from build123d import *

# Parameters (mm, degrees)
FACE_2_DEPTH            = 5
SKETCH2_W               = 14.632926246
SKETCH2_H               = 5
BOSS_EXTRUDE2_DEPTH     = 7
SKETCH3_W               = 14.632926246
SKETCH3_H               = 7
BOSS_EXTRUDE3_DEPTH     = 7
EYE_HOLES_REACH         = 248.075
SKETCH4_R               = 1.15
SKETCH5_W               = 14.632926246
SKETCH5_H               = 3.5
SEAT_DEPTH              = 7
SKETCH6_W               = 18
SKETCH6_H               = 5
BOSS_EXTRUDE4_DEPTH     = 3.5
SKETCH7_W               = 18.025006546
SKETCH7_H               = 4.25
TOP_HOLE_DEPTH          = 248.972829901
MIDDLE_HOLE_DEPTH       = 246.672789516
MIDDLE_HOLE_DEPTH_BACK  = 246.672789516
SKETCH8_R               = 5.003684601
CUT_EXTRUDE8_DEPTH      = 208.598432106
CUT_EXTRUDE8_DEPTH_BACK = 3.5
SKETCH10_R              = 1.15
SKETCH11_R              = 0.754398486
CUT_EXTRUDE9_DEPTH      = 246.672789516


with BuildPart() as part:
    # Sketch1 → Face 2 (new body)
    with BuildSketch(Plane.XY):
        Polygon((189.199131389, 129.336090234), (189.219408928, 129.168352428), (189.276625012, 129.01501095), (189.375109043, 128.870497126), (189.879763338, 128.333185306), (190.417075159, 127.828531011), (190.558185088, 127.731803407), (190.715733881, 127.672634267), (190.882668266, 127.652553357), (205.515594512, 127.652553357), (205.683332318, 127.672830896), (205.84007769, 127.731803407), (205.98118762, 127.828531011), (207.023153735, 128.870497126), (207.118523911, 129.009007135), (207.17885385, 129.168352428), (207.199131389, 129.336090234), (207.199131389, 132.202042434), (189.199131389, 132.202042434), align=None)
    extrude(amount=FACE_2_DEPTH)

    # Sketch2 → Boss-Extrude2 (add)
    with BuildSketch(Plane.XZ.offset(-127.652553357)):
        with Locations((198.199131389, 2.5)):
            Rectangle(SKETCH2_W, SKETCH2_H)
    extrude(amount=BOSS_EXTRUDE2_DEPTH)

    # Sketch3 → Boss-Extrude3 (add)
    with BuildSketch(Plane(origin=(0, 0, 0), x_dir=(-1, 0, 0), z_dir=(0, 0, -1))):
        with Locations((-198.199131389, 124.152553357)):
            Rectangle(SKETCH3_W, SKETCH3_H)
    extrude(amount=BOSS_EXTRUDE3_DEPTH)

    # Sketch4 → Eye Holes (cut, up to next)
    with BuildSketch(Plane.XY.offset(5), mode=Mode.PRIVATE) as eye_holes_sk1:
        with Locations((191.649131389, 129.852042434)):
            Circle(SKETCH4_R)
    eye_holes_tool1 = extrude(eye_holes_sk1.sketch, amount=-EYE_HOLES_REACH, mode=Mode.PRIVATE) & part.part
    # Sketch4 → Eye Holes (cut, up to next)
    with BuildSketch(Plane.XY.offset(5), mode=Mode.PRIVATE) as eye_holes_sk2:
        with Locations((204.599131389, 129.852042434)):
            Circle(SKETCH4_R)
    eye_holes_tool2 = extrude(eye_holes_sk2.sketch, amount=-EYE_HOLES_REACH, mode=Mode.PRIVATE) & part.part
    add(eye_holes_tool1.solids().sort_by_distance((191.649131, 129.852042, 5))[0], mode=Mode.SUBTRACT)
    add(eye_holes_tool2.solids().sort_by_distance((204.599131, 129.852042, 5))[0], mode=Mode.SUBTRACT)

    # Sketch5 → Seat (cut)
    with BuildSketch(Plane(origin=(0, 0, -7), x_dir=(-1, 0, 0), z_dir=(0, 0, -1))):
        with Locations((-198.199131389, 125.902553357)):
            Rectangle(SKETCH5_W, SKETCH5_H)
    extrude(amount=-SEAT_DEPTH, mode=Mode.SUBTRACT)

    # Sketch6 → Boss-Extrude4 (add)
    with BuildSketch(Plane(origin=(0, 132.202042434, 0), x_dir=(1, 0, 0), z_dir=(0, 1, 0))):
        with Locations((198.199131389, -2.5)):
            Rectangle(SKETCH6_W, SKETCH6_H)
    extrude(amount=BOSS_EXTRUDE4_DEPTH)

    # Sketch7 → Top Hole (cut, through all)
    with BuildSketch(Plane.XY.offset(5)):
        with Locations((198.194207579, 133.577042434)):
            Rectangle(SKETCH7_W, SKETCH7_H)
    extrude(amount=-TOP_HOLE_DEPTH, mode=Mode.SUBTRACT)

    # Sketch8 → Middle Hole (cut, two sides: drawn at the far end of the back side and taken through both)
    with BuildSketch(Plane.XY.offset(5).offset(-MIDDLE_HOLE_DEPTH_BACK)):
        with Locations((198.199131389, 131.452042434)):
            Circle(SKETCH8_R)
    extrude(amount=MIDDLE_HOLE_DEPTH + MIDDLE_HOLE_DEPTH_BACK, mode=Mode.SUBTRACT)

    # Sketch10 → Cut-Extrude8 (cut, two sides: drawn at the far end of the back side and taken through both)
    with BuildSketch(Plane.XZ.offset(-120.652553357).offset(-CUT_EXTRUDE8_DEPTH_BACK)):
        with Locations((193.382668266, -3.308334882)):
            Circle(SKETCH10_R)
        with Locations((203.015594512, -3.308334882)):
            Circle(SKETCH10_R)
    extrude(amount=CUT_EXTRUDE8_DEPTH + CUT_EXTRUDE8_DEPTH_BACK, mode=Mode.SUBTRACT)

    # Sketch11 → Cut-Extrude9 (cut, through all)
    with BuildSketch(Plane.XY.offset(5)):
        with Locations((192.88691871, 131.452042434)):
            Circle(SKETCH11_R)
        with Locations((202.919958348, 131.377258625)):
            Circle(SKETCH11_R)
    extrude(amount=-CUT_EXTRUDE9_DEPTH, mode=Mode.SUBTRACT)


solid = part.part
Could you check a few things on this model? Use its own coordinates, in mm. A direction names the side the tool comes from. Coordinates: 2 decimals unless noted, no trailing zeros. Order: outer loops, then holes, each group sorted by start corner. A loop starts at its lowest first (then second) coordinate and runs counter-clockwise, first axis right, second up.
Q1. Suppose I cut it at A-A on x = 191.25. Please give me the cut outline in (y, z).
Q2. Which directions (+Z, -Z, +X, -X, +Y, -Y) give clear straight access to the entire face, cutting with the end or side of a thin tool? Please do faces 5 (the flat face through (198, 126, 0)), 6 (the flat face through (190.883, 123, 0)), 7 (the cylindrical face through (192.234, 122.427, -3.258)), 8 (the flat face through (205.516, 123, 0)).
Q3. Will these pins go through, and if not, where does the flat tip stop? pin 1 (2 mm diameter, centred on x = 193.38, z = -3.31, fed in from +Y); pin 2 (3.5 mm diameter, centred on y = 122.5, z = -3, fed in from -X); pin 3 (3.5 mm diameter, centred on x = 203.02, z = -3.31, fed in from +Y); pin 4 (2 mm diameter, centred on y = 127.5, z = 3, fed in from +X).
Q4. Suppose I cut it at D-D on y = 123.5. Please give me the cut outline in (x, z).
Q5. Please list where these lines run through material, in increasing order: L1, parallel to Y at x = 195.75, z = -6; L2, parallel to X at y = 124.5, z = 4.5; L3, parallel to Z at x = 194, y = 127.75.
Q6. Suppose I cut it at B-B on z = 3.75. Please give me the cut outline in (x, y).
Q7. Suppose I cut it at C-C on z = -4.75. Please give me the cut outline in (x, y).
Q8. Thinking about a two-plate mould opening in Y: for faces 1 (the flat face through (198, 122, -7)), 2 (the flat face through (191, 131.452, 3)), 3 (the cylindrical face through (190.8, 130.63, 2.54)), 4 (the cylindrical face through (204.449, 130.992, 2.535)), which applies, released by +Y, released by -Y, zero draft, split by the parting line, or undercut?
Answer:
1. outline: (120.65, -7) - (124.15, -7) - (124.15, 0) - (128.77, 0) - (128.77, 5) - (120.65, 5) - close; (130.93, 0) - (131.45, 0) - (131.45, 5) - (130.93, 5) - close
2. face 5: -Z, +X, -X, +Y
2. face 6: +Z, -Z, -X, -Y
2. face 7: +Y, -Y
2. face 8: +Z, -Z, +X, -Y
3. pin 1: passes through
3. pin 2: stops at x = 190.88
3. pin 3: stops at y = 124.15
3. pin 4: stops at x = 206.65
4. outline: (190.88, -7) - (205.52, -7) - (205.52, 5) - (190.88, 5) - close; hole circle Ø2.3 at (193.38, -3.31); hole circle Ø2.3 at (203.02, -3.31)
5. L1: y = 120.65 to 124.15
5. L2: x = 190.88 to 205.52
5. L3: z = 0 to 5
6. outline: (189.2, 129.34) - (189.22, 129.17) - (189.28, 129.02) - (189.38, 128.87) - (189.88, 128.33) - (190.42, 127.83) - (190.56, 127.73) - (190.72, 127.67) - (190.88, 127.65) - (190.88, 120.65) - (205.52, 120.65) - (205.52, 127.65) - (205.68, 127.67) - (205.84, 127.73) - (205.98, 127.83) - (207.02, 128.87) - (207.12, 129.01) - (207.18, 129.17) - (207.2, 129.34) - (207.2, 131.45) - (203.67, 131.45) arc R0.75 cw to (203.14, 130.66) arc R5 cw to (193.24, 130.79) arc R0.75 cw to (192.13, 131.45) - (189.2, 131.45) - close; hole circle Ø2.3 at (191.65, 129.85); hole circle Ø2.3 at (204.6, 129.85)
7. outline: (190.88, 120.65) - (205.52, 120.65) - (205.52, 124.15) - (190.88, 124.15) - close
8. face 1: zero draft
8. face 2: released by +Y
8. face 3: undercut
8. face 4: undercut
